Design review of the part built by this model. Coordinates are the model's own, in mm. Face numbers are marked on the shaded views. A direction names the side the tool comes from. Coordinates: 2 decimals unless noted, no trailing zeros. Write each loop counter-clockwise with the first axis right and the second up, starting at its lowest first coordinate (ties: lowest second). Pieces come first, ordered by that corner, then holes. Notation, with made-up numbers: (62.25, -4) -> (97.25, -4) arc R24 cw to (97.25, 27) -> close; hole circle Ø9 at (2.5, 29). An arc over 180 degrees is marked (long way). Answer in a Markdown table with one row per item. Add a question column.
Item 1: To check wall thickness, follow line 1 (X direction, y = 0.85, z = -8.25); line 2 (X direction, y = 13, z = -4.5); line 3 (X direction, y = 1.75, z = 12). State the ranges of each line that lie inside material, in increasing order.
Item 2: Take a section at D-D, the plane y = 1.5. Give the number of separate pieces and of enclosed holes in the cut face, and give its area (3 significant figures).
Item 3: Take a section at B-B, the plane x = -46. Write out the cut boundary in (y, z).
Item 4: Take a section at C-C, the plane y = 12.5. Write out the cut boundary in (x, z).
Item 5: Take a section at A-A, the plane z = 37. Write out the cut boundary in (x, y).
Item 6: Clearance check with flat-ended pins moving along their axes: P1, Ø4.5, axis at x = 28.5, z = 41, coming from the +Y side; P2, Ø0.8, axis at y = 9.5, z = 26, coming from the +X side; P3, Ø5, axis at y = 14, z = -19, coming from the -X side. State where each tip first meets the part, or that it passes through.
Item 7: Draft analysis for pull direction X (two halves, no side actions). For the marked faces 3, 4 and 5, state which applies: released by +X, released by -X, zero draft, split by the parting line, or undercut.
Item 8: For the marked faces 1 and 2, list the 3-axis set-ups (+Z, -Z, +X, -X, +Y, -Y) from which the entire face can be reached by the end or side of a thin tool; tool diameter is ignored.
from build123d import *

# Parameters (mm, degrees)
SKETCH_1_R          = 1.75
EXTRUDE_1_DEPTH     = 3
EXTRUDE_2_DEPTH     = 11
EXTRUDE_3_DEPTH     = 1.5
SKETCH_5_R          = 10
CUT_EXTRUDE_1_DEPTH = 81.562087858
SKETCH_6_R          = 5
CUT_EXTRUDE_2_DEPTH = 5
SKETCH_7_R          = 5
CUT_EXTRUDE_3_DEPTH = 5
CUT_EXTRUDE_4_DEPTH = 3


with BuildPart() as part:
    # 草图1 → 凸台-拉伸1 (new body)
    with BuildSketch(Plane(origin=(0, 0, 0), x_dir=(1, 0, 0), z_dir=(0, 1, 0))):
        with BuildLine():
            Line((-60, 45), (60, 45))
            ThreePointArc((60, 45), (63.535533906, 43.535533906), (65, 40))
            Line((65, 40), (65, -40))
            ThreePointArc((65, -40), (63.535533906, -43.535533906), (60, -45))
            Line((60, -45), (-60, -45))
            ThreePointArc((-60, -45), (-63.535533906, -43.535533906), (-65, -40))
            Line((-65, -40), (-65, 40))
            ThreePointArc((-65, 40), (-63.535533906, 43.535533906), (-60, 45))
        make_face()
        with Locations(Location((-60, 8.25, 0), (0, 0, 270))):
            Circle(SKETCH_1_R, mode=Mode.SUBTRACT)
        with Locations(Location((-46, 8.25, 0), (0, 0, 270))):
            Circle(SKETCH_1_R, mode=Mode.SUBTRACT)
        with Locations(Location((-46, -8.25, 0), (0, 0, 90))):
            Circle(SKETCH_1_R, mode=Mode.SUBTRACT)
        with Locations(Location((-60, -8.25, 0), (0, 0, 90))):
            Circle(SKETCH_1_R, mode=Mode.SUBTRACT)
        with Locations(Location((60, 8.25, 0), (0, 0, 90))):
            Circle(SKETCH_1_R, mode=Mode.SUBTRACT)
        with Locations(Location((60, -8.25, 0), (0, 0, 270))):
            Circle(SKETCH_1_R, mode=Mode.SUBTRACT)
        with Locations(Location((46, -8.25, 0), (0, 0, 270))):
            Circle(SKETCH_1_R, mode=Mode.SUBTRACT)
        with Locations(Location((46, 8.25, 0), (0, 0, 90))):
            Circle(SKETCH_1_R, mode=Mode.SUBTRACT)
        with Locations(Location((-28.5, 41, 0), (0, 0, 270))):
            Circle(SKETCH_1_R, mode=Mode.SUBTRACT)
        with Locations(Location((-28.5, -41, 0), (0, 0, 90))):
            Circle(SKETCH_1_R, mode=Mode.SUBTRACT)
        with Locations(Location((28.5, -41, 0), (0, 0, 270))):
            Circle(SKETCH_1_R, mode=Mode.SUBTRACT)
        with Locations(Location((28.5, 41, 0), (0, 0, 90))):
            Circle(SKETCH_1_R, mode=Mode.SUBTRACT)
    extrude(amount=EXTRUDE_1_DEPTH)

    # 草图2 → 凸台-拉伸2 (add)
    with BuildSketch(Plane(origin=(0, 3, 0), x_dir=(1, 0, 0), z_dir=(0, 1, 0))):
        Polygon((18, 25.5), (19.5, 25.5), (19.5, -27), (-19.5, -27), (-19.5, 25.5), (-18, 25.5), (-18, -25.5), (18, -25.5), align=None)
    extrude(amount=EXTRUDE_2_DEPTH)

    # 草图3 → 凸台-拉伸3 (add)
    with BuildSketch(Plane(origin=(0, 14, 0), x_dir=(1, 0, 0), z_dir=(0, 1, 0))):
        with BuildLine():
            Line((-15, 24), (-18, 24))
            Line((-18, 24), (-18, -25.5))
            Line((-18, -25.5), (18, -25.5))
            Line((18, -25.5), (18, 24))
            Line((18, 24), (15, 24))
            ThreePointArc((15, 24), (0, 9), (-15, 24))
        make_face()
        Polygon((-18, 24), (-19.5, 24), (-19.5, -27), (19.5, -27), (19.5, 24), (18, 24), (18, -25.5), (-18, -25.5), align=None)
    extrude(amount=EXTRUDE_3_DEPTH)

    # 草图5 → 切除-拉伸1 (cut, through all)
    with BuildSketch(Plane(origin=(0, 15.5, 0), x_dir=(1, 0, 0), z_dir=(0, 1, 0))):
        with Locations(Location((0, -12, 0), (0, 0, 270))):
            Circle(SKETCH_5_R)
    extrude(amount=-CUT_EXTRUDE_1_DEPTH, mode=Mode.SUBTRACT)

    # 草图6 → 切除-拉伸2 (cut)
    with BuildSketch(Plane(origin=(19.5, 0, 0), x_dir=(0, 0, -1), z_dir=(1, 0, 0))):
        with Locations((-27, 9.25)):
            Circle(SKETCH_6_R)
    cut_extrude_2 = extrude(amount=-CUT_EXTRUDE_2_DEPTH, mode=Mode.SUBTRACT)

    # 草图7 → 切除-拉伸3 (cut)
    with BuildSketch(Plane.XY.offset(27)):
        with Locations((19.5, 9.25)):
            Circle(SKETCH_7_R)
    cut_extrude_3 = extrude(amount=-CUT_EXTRUDE_3_DEPTH, mode=Mode.SUBTRACT)

    # 镜向1: 切除-拉伸2, 切除-拉伸3 across plane
    add(cut_extrude_2.mirror(Plane(origin=(0, 0, 0), x_dir=(0, 0, 1), z_dir=(1, 0, 0))), mode=Mode.SUBTRACT)
    add(cut_extrude_3.mirror(Plane(origin=(0, 0, 0), x_dir=(0, 0, 1), z_dir=(1, 0, 0))), mode=Mode.SUBTRACT)

    # 草图8 → 切除-拉伸4 (cut)
    with BuildSketch(Plane(origin=(0, 3, 0), x_dir=(1, 0, 0), z_dir=(0, 1, 0))):
        with BuildLine():
            Line((-17.5, -34), (17.5, -34))
            ThreePointArc((17.5, -34), (20.5, -37), (17.5, -40))
            Line((17.5, -40), (-17.5, -40))
            ThreePointArc((-17.5, -40), (-20.5, -37), (-17.5, -34))
        make_face()
    cut_extrude_4 = extrude(amount=-CUT_EXTRUDE_4_DEPTH, mode=Mode.SUBTRACT)

    # 镜向2: 切除-拉伸4 across plane
    add(cut_extrude_4.mirror(Plane.XY), mode=Mode.SUBTRACT)


solid = part.part
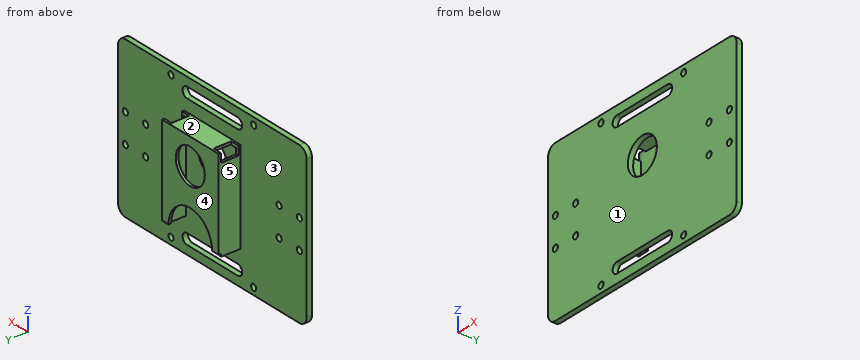
Answers:
| question | item | result |
|---|---|---|
| 1 | line 1 | x = -65 to -61.75, -58.25 to -47.75, -44.25 to 44.25, 47.75 to 58.25, 61.75 to 65 |
| 1 | line 2 | x = -19.5 to -18, 18 to 19.5 |
| 1 | line 3 | x = -65 to -10, 10 to 65 |
| 2 | separate pieces | 1 |
| 2 | enclosed holes | 15 |
| 2 | area | 10,800 mm^2 |
| 3 | outline | (0, -45) -> (3, -45) -> (3, -10) -> (0, -10) -> close; (0, -6.5) -> (3, -6.5) -> (3, 6.5) -> (0, 6.5) -> close; (0, 10) -> (3, 10) -> (3, 45) -> (0, 45) -> close |
| 4 | outline | (-19.5, -25.5) -> (-18, -25.5) -> (-18, 22) -> (-19.5, 22) -> close; (-14.5, 25.5) -> (14.5, 25.5) -> (14.5, 27) -> (-14.5, 27) -> close; (18, -25.5) -> (19.5, -25.5) -> (19.5, 22) -> (18, 22) -> close |
| 5 | outline | (-65, 0) -> (-20.5, 0) -> (-20.5, 3) -> (-65, 3) -> close; (20.5, 0) -> (65, 0) -> (65, 3) -> (20.5, 3) -> close |
| 6 | P1 | stops at y = 3 |
| 6 | P2 | stops at x = 14.5 |
| 6 | P3 | stops at x = -19.5 |
| 7 | face 3 | undercut |
| 7 | face 4 | zero draft |
| 7 | face 5 | released by -X |
| 8 | face 1 | +Z, -Z, +X, -X, -Y |
| 8 | face 2 | +Z, +X, -X, +Y |
